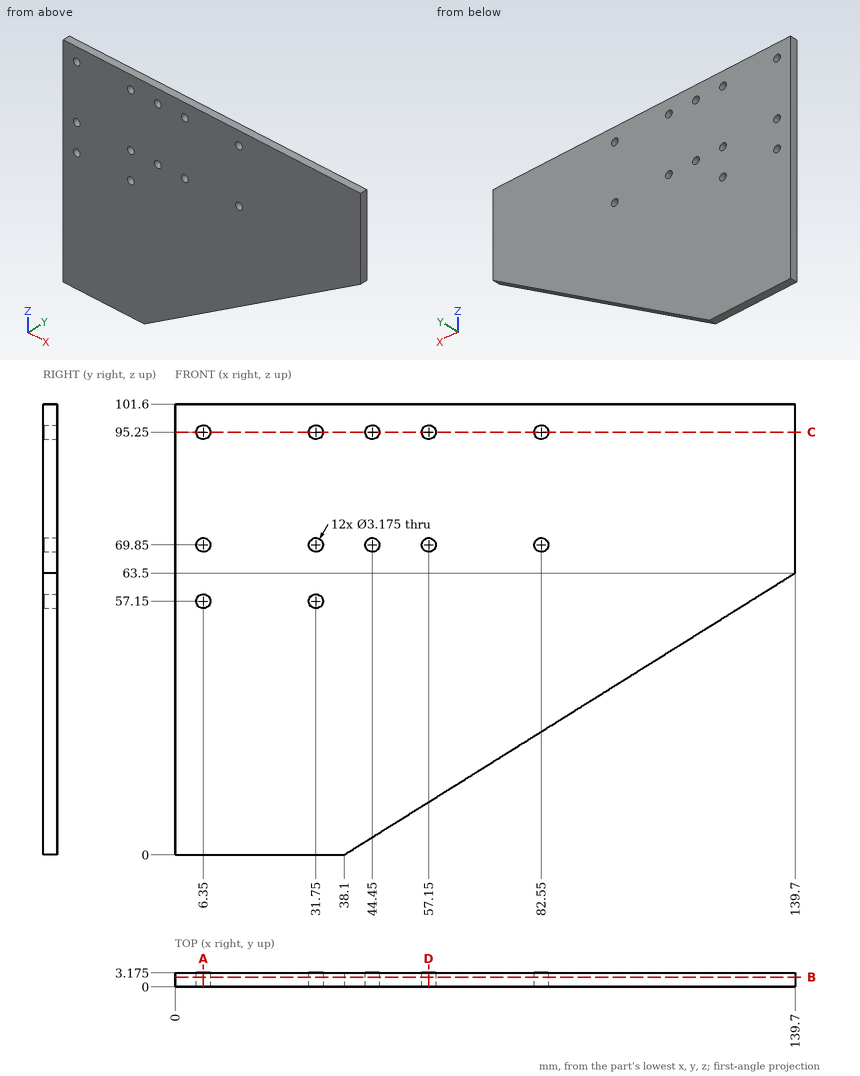
Job drawing, mm, ordinate dimensions from the low corner. One solid piece. Coordinates: 2 decimals unless noted, no trailing zeros. Order: outer loops, then holes, each group sorted by start corner. A loop starts at its lowest first (then second) coordinate and runs counter-clockwise, first axis right, second up. Notation, with made-up numbers: M 60.5,62.25 L 98.5,62.25 A11 ccw 98.5,72.25 Z; hole C 10.5,57 d3. An arc over 180 degrees is marked long. Return JSON: item names as keys, results as strings.
1. Flat gauge pin, fed straight in: pin 1 (2.5 mm diameter, centred on x = 6.35, z = 69.85, fed in from +Y). Where does the tip first touch, or does it go through?
Ans:
{"pin 1": "through"}
2. Saw through at C-C (z = 95.25). Give the cut face in (x, y) (1 decimal), and give its area (3 significant figures).
Ans:
{"outline": "M 0,0 L 4.8,0 L 4.8,3.2 L 0,3.2 Z; M 7.9,0 L 30.2,0 L 30.2,3.2 L 7.9,3.2 Z; M 33.3,0 L 42.9,0 L 42.9,3.2 L 33.3,3.2 Z; M 46,0 L 55.6,0 L 55.6,3.2 L 46,3.2 Z; M 58.7,0 L 81,0 L 81,3.2 L 58.7,3.2 Z; M 84.1,0 L 139.7,0 L 139.7,3.2 L 84.1,3.2 Z", "area": "393 mm^2"}
3. Saw through at B-B (y = 2.2). Give the number of separate pieces and of enclosed holes in the cut face, and give its area (3 significant figures).
Ans:
{"separate pieces": "1", "enclosed holes": "12", "area": "10,900 mm^2"}
4. Saw through at A-A (x = 6.35). Give the cut face in (y, z) (1 decimal), and give its area (3 significant figures).
Ans:
{"outline": "M 0,0 L 3.2,0 L 3.2,55.6 L 0,55.6 Z; M 0,58.7 L 3.2,58.7 L 3.2,68.3 L 0,68.3 Z; M 0,71.4 L 3.2,71.4 L 3.2,93.7 L 0,93.7 Z; M 0,96.8 L 3.2,96.8 L 3.2,101.6 L 0,101.6 Z", "area": "292 mm^2"}
5. Drill centre lines: probe 1 along Z at (x, y) = (31.75, 1.4); probe 2 along X at (y, z) = (0.8, 95.25); probe 3 along Z at (x, y) = (57, 1.5). Where is each one in solid material? Low to high.
Ans:
{"probe 1": "0 to 55.56, 58.74 to 68.26, 71.44 to 93.66, 96.84 to 101.6", "probe 2": "0 to 4.76, 7.94 to 30.16, 33.34 to 42.86, 46.04 to 55.56, 58.74 to 80.96, 84.14 to 139.7", "probe 3": "11.81 to 68.27, 71.43 to 93.67, 96.83 to 101.6"}
6. Saw through at D-D (x = 57.15). Give the cut face in (y, z) (1 decimal).
Ans:
{"outline": "M 0,11.9 L 3.2,11.9 L 3.2,68.3 L 0,68.3 Z; M 0,71.4 L 3.2,71.4 L 3.2,93.7 L 0,93.7 Z; M 0,96.8 L 3.2,96.8 L 3.2,101.6 L 0,101.6 Z"}
